Geometry check sheet. Reference: drawing and pictorial views, mm from the part's lowest x, y, z. A direction names the side the tool comes from. Coordinates: 2 decimals unless noted, no trailing zeros. Loops run counter-clockwise (first coordinate to the right, second up) from the corner with the lowest first, then second, coordinate; pieces in that order, holes last. Notation, with made-up numbers: (0, -5) -> (36, -5) arc R11 ccw to (36, 14) -> close; hole circle Ø9 at (34, 82.25). An arc over 180 degrees is marked (long way). Answer as a JSON object with one key per item and string values.
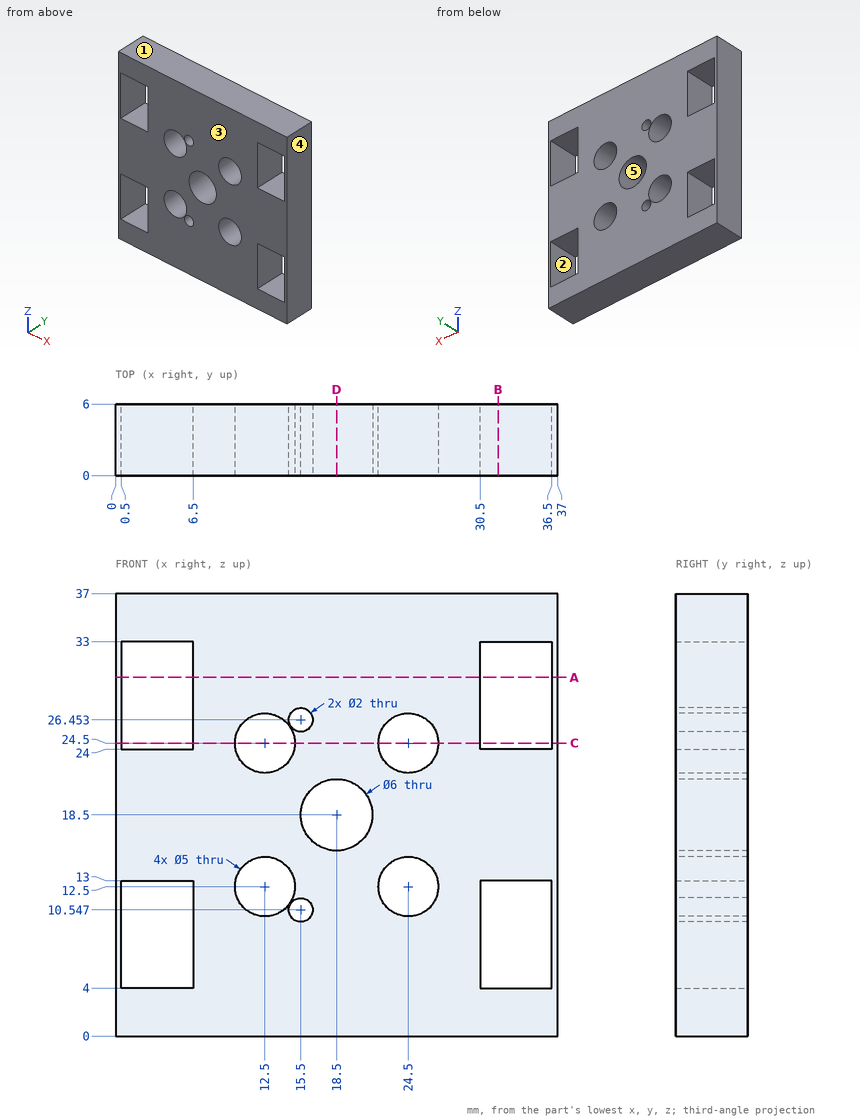
1. Section check D-D, the plane x = 18.5. Record the boundary of the cut face in (y, z), then the cut area to 3 significant figures.
Evaluation:
{"outline": "(0, 0) -> (6, 0) -> (6, 15.5) -> (0, 15.5) -> close; (0, 21.5) -> (6, 21.5) -> (6, 37) -> (0, 37) -> close", "area": "186 mm^2"}
2. Mould release check, pull along X, two halves, no side actions. Record for the marked faces 3, 4 and 5: released by +X, released by -X, zero draft, split by the parting line, or undercut.
Evaluation:
{"face 3": "zero draft", "face 4": "released by +X", "face 5": "undercut"}
3. Section check A-A, the plane z = 30. Record the boundary of the cut face in (x, y), then the cut area to 3 significant figures.
Evaluation:
{"outline": "(0, 0) -> (0.5, 0) -> (0.5, 6) -> (0, 6) -> close; (6.5, 0) -> (30.5, 0) -> (30.5, 6) -> (6.5, 6) -> close; (36.5, 0) -> (37, 0) -> (37, 6) -> (36.5, 6) -> close", "area": "150 mm^2"}
4. Section check C-C, the plane z = 24.5. Record the boundary of the cut face in (x, y).
Evaluation:
{"outline": "(0, 0) -> (0.5, 0) -> (0.5, 6) -> (0, 6) -> close; (6.5, 0) -> (10, 0) -> (10, 6) -> (6.5, 6) -> close; (15, 0) -> (22, 0) -> (22, 6) -> (15, 6) -> close; (27, 0) -> (30.5, 0) -> (30.5, 6) -> (27, 6) -> close; (36.5, 0) -> (37, 0) -> (37, 6) -> (36.5, 6) -> close"}
5. Tool access check on the marked faces 1 and 2. Record the directions out of +Z, -Z, +X, -X, +Y, -Y that give a thin tool (end or side, any length) a straight path to the whole face; none if there is none.
Evaluation:
{"face 1": "+Z, +X, -X, +Y, -Y", "face 2": "+Y, -Y"}
6. Thickness scan on probe 1 along Z at (x, y) = (18.5, 3.25); probe 2 along Z at (x, y) = (6, 4.1); probe 3 along Z at (x, y) = (12.5, 4). Record the ranges inside material, lowest first. Write a range as from..to.
Evaluation:
{"probe 1": "z = 0..15.5, 21.5..37", "probe 2": "z = 0..4, 13..24, 33..37", "probe 3": "z = 0..10, 15..22, 27..37"}
7. Section check B-B, the plane x = 32. Record the boundary of the cut face in (y, z).
Evaluation:
{"outline": "(0, 0) -> (6, 0) -> (6, 4) -> (0, 4) -> close; (0, 13) -> (6, 13) -> (6, 24) -> (0, 24) -> close; (0, 33) -> (6, 33) -> (6, 37) -> (0, 37) -> close"}
